Geometry check sheet. Reference: drawing and pictorial views, mm from the part's lowest x, y, z. Coordinates: 2 decimals unless noted, no trailing zeros. Write each loop counter-clockwise with the first axis right and the second up, starting at its lowest first coordinate (ties: lowest second). Pieces come first, ordered by that corner, then holes. Notation, with made-up numbers: (37.25, 18.25) -> (73.25, 18.25) arc R18 ccw to (73.25, 50.25) -> close; hole circle Ø1 at (40, -29). An arc over 180 degrees is marked (long way). Put each result on its own line as item: value.
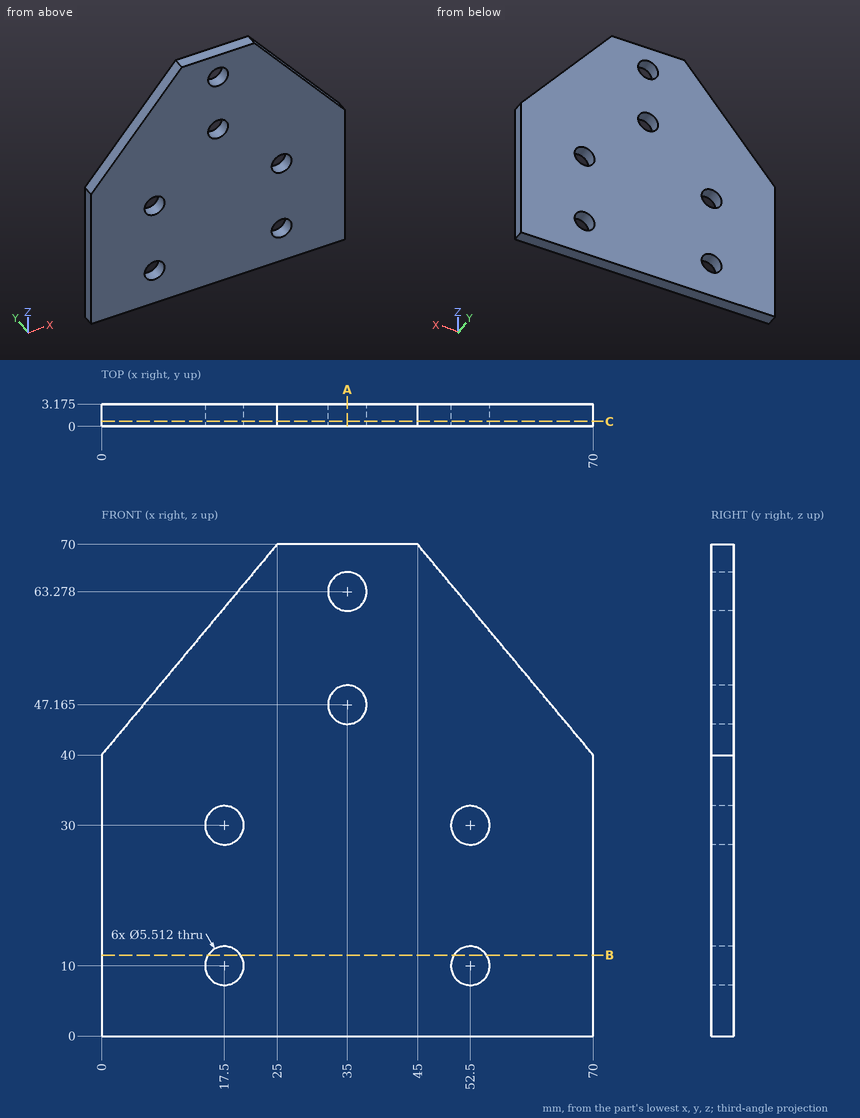
Q1. Cross-section at B-B (z = 11.5). Record the cut outline in (x, y) (1 decimal), plus the area to 3 significant figures.
Recorded:
outline: (0, 0) -> (15.2, 0) -> (15.2, 3.2) -> (0, 3.2) -> close; (19.8, 0) -> (50.2, 0) -> (50.2, 3.2) -> (19.8, 3.2) -> close; (54.8, 0) -> (70, 0) -> (70, 3.2) -> (54.8, 3.2) -> close
area: 193 mm2
Q2. Material ranges on line 1 along Z through (x, y) = (35, 1.2) (1 decimal); line 2 along Z through (x, y) = (17.5, 1) (1 decimal); line 3 along X through (y, z) = (1.8, 10.5), recorded low to high.
Recorded:
line 1: z = 0 to 44.4, 49.9 to 60.5, 66 to 70
line 2: z = 0 to 7.2, 12.8 to 27.2, 32.8 to 61
line 3: x = 0 to 14.79, 20.21 to 49.79, 55.21 to 70
Q3. Cross-section at A-A (x = 35). Record the cut outline in (y, z) (1 decimal), plus the area to 3 significant figures.
Recorded:
outline: (0, 0) -> (3.2, 0) -> (3.2, 44.4) -> (0, 44.4) -> close; (0, 49.9) -> (3.2, 49.9) -> (3.2, 60.5) -> (0, 60.5) -> close; (0, 66) -> (3.2, 66) -> (3.2, 70) -> (0, 70) -> close
area: 187 mm2
Q4. Depth check by flat-ended pin: P1, Ø4.5, axis at x = 52.5, z = 10, coming from the +Y side. Enter the tip coordinate at first touch or a pass-through.
Recorded:
P1: passes through
Q5. Cross-section at C-C (y = 0.7). Record the cut outline in (x, z) (1 decimal).
Recorded:
outline: (0, 0) -> (70, 0) -> (70, 40) -> (45, 70) -> (25, 70) -> (0, 40) -> close; hole circle Ø5.5 at (17.5, 10); hole circle Ø5.5 at (17.5, 30); hole circle Ø5.5 at (35, 47.2); hole circle Ø5.5 at (35, 63.3); hole circle Ø5.5 at (52.5, 10); hole circle Ø5.5 at (52.5, 30)
